Can you work these out from the model? Positions are in its coordinate system, mm. Give positions to 0.01 mm unless a question says otherwise; leave off trailing zeros. Loops run counter-clockwise (first coordinate to the right, second up) from the corner with the lowest first, then second, coordinate; pieces in that order, holes last.
from build123d import *

# Parameters (mm, degrees)
SKETCH_1_R      = 1.5
SKETCH_1_R_2    = 11.05
EXTRUDE_1_DEPTH = 2


with BuildPart() as part:
    # 草图1 → 凸台-拉伸1 (new body)
    with BuildSketch(Plane.XY):
        with BuildLine():
            Line((-2.598076211, 21.5), (-19.918584287, -8.5))
            ThreePointArc((-19.918584287, -8.5), (-19.918584287, -11.5), (-17.320508076, -13))
            Line((-17.320508076, -13), (17.320508076, -13))
            ThreePointArc((17.320508076, -13), (19.918584287, -11.5), (19.918584287, -8.5))
            Line((19.918584287, -8.5), (2.598076211, 21.5))
            ThreePointArc((2.598076211, 21.5), (0, 23), (-2.598076211, 21.5))
        make_face()
        with Locations((-17.320508076, -10)):
            Circle(SKETCH_1_R, mode=Mode.SUBTRACT)
        with Locations((0, 20)):
            Circle(SKETCH_1_R, mode=Mode.SUBTRACT)
        with Locations((17.320508076, -10)):
            Circle(SKETCH_1_R, mode=Mode.SUBTRACT)
        Circle(SKETCH_1_R_2, mode=Mode.SUBTRACT)
    extrude(amount=EXTRUDE_1_DEPTH)


solid = part.part
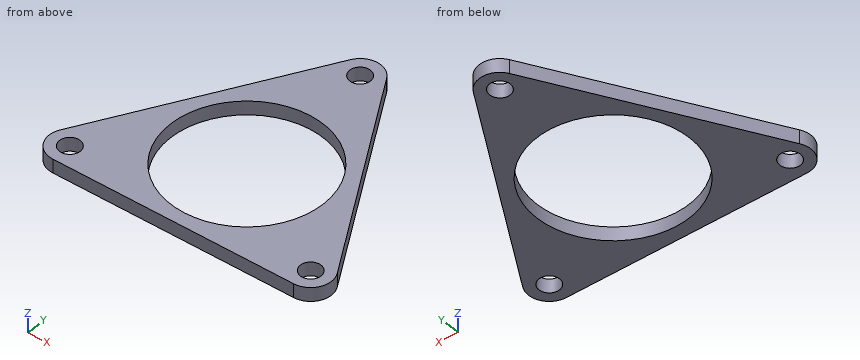
(1) Suppose I cut it at B-B on x = -5. List the corners of the cut face in (y, z) for me, plus the area to 3 significant figures.
Returned:
outline: (-13, 0) - (-9.85, 0) - (-9.85, 2) - (-13, 2) - close; (9.85, 0) - (17.34, 0) - (17.34, 2) - (9.85, 2) - close
area: 21.3 mm2
(2) Suppose I cut it at D-D on y = 0. List the corners of the cut face in (x, z) for me.
Returned:
outline: (-15.01, 0) - (-11.05, 0) - (-11.05, 2) - (-15.01, 2) - close; (11.05, 0) - (15.01, 0) - (15.01, 2) - (11.05, 2) - close
(3) Suppose I cut it at C-C on z = 1.6. List the corners of the cut face in (x, y) for me, plus the area to 3 significant figures.
Returned:
outline: (-19.92, -8.5) arc R3 ccw to (-17.32, -13) - (17.32, -13) arc R3 ccw to (19.92, -8.5) - (2.6, 21.5) arc R3 ccw to (-2.6, 21.5) - close; hole circle Ø3 at (-17.32, -10); hole circle Ø22.1 at (0, 0); hole circle Ø3 at (0, 20); hole circle Ø3 at (17.32, -10)
area: 455 mm2
(4) Please list where these lines run through material, in increasing order: probe 1 along Y at (x, z) = (0, 0.7); probe 2 along X at (y, z) = (-9, 1.65); probe 3 along Y at (x, z) = (-6, 1.3).
Returned:
probe 1: y = -13 to -11.05, 11.05 to 18.5, 21.5 to 23
probe 2: x = -20.15 to -18.44, -16.2 to -6.41, 6.41 to 16.2, 18.44 to 20.15
probe 3: y = -13 to -9.28, 9.28 to 15.61
(5) Suppose I cut it at A-A on x = 0. List the corners of the cut face in (y, z) for me.
Returned:
outline: (-13, 0) - (-11.05, 0) - (-11.05, 2) - (-13, 2) - close; (11.05, 0) - (18.5, 0) - (18.5, 2) - (11.05, 2) - close; (21.5, 0) - (23, 0) - (23, 2) - (21.5, 2) - close
(6) Will these pins go through, and if not, where does the flat tip stop? P1, Ø5, axis at x = -9.5, y = 17, coming from the -Z side; P2, Ø1, axis at y = 9, z = 0.5, coming from the +X side; P3, Ø1, axis at y = 17, z = 1, coming from the -X side; P4, Ø1, axis at y = -4.5, z = 0.5, coming from the -X side.
Returned:
P1: passes through
P2: stops at x = 10.1
P3: stops at x = -5.48
P4: stops at x = -17.9
